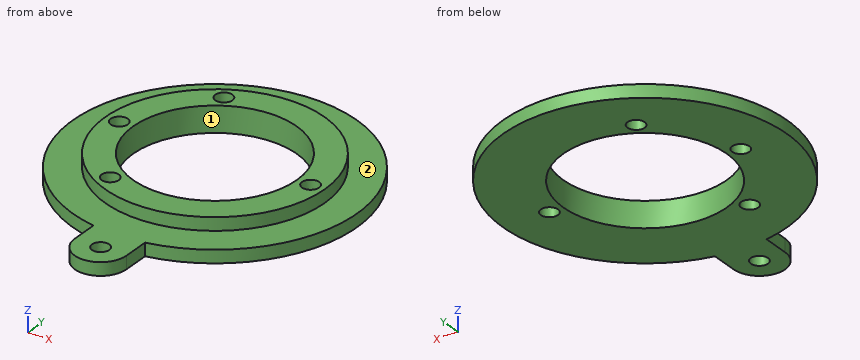
```python
from build123d import *

# Parameters (mm, degrees)
SKETCH010_R     = 25.5
SKETCH010_R_2   = 19
PAD005_DEPTH    = 3
SKETCH011_R     = 19
SKETCH011_R_2   = 2
PAD006_DEPTH    = 3
SKETCH012_R     = 2
POCKET002_DEPTH = 6.001


with BuildPart() as part:
    # Sketch010 → Pad005 (new body)
    with BuildSketch(Plane.XY):
        Circle(SKETCH010_R)
        Circle(SKETCH010_R_2, mode=Mode.SUBTRACT)
    extrude(amount=PAD005_DEPTH)

    # Sketch011 (on Face3 of Pad005) → Pad006 (join)
    with BuildSketch(Plane(origin=(0, 0, 0), x_dir=(1, 0, 0), z_dir=(0, 0, -1))):
        with BuildLine():
            ThreePointArc((-6, 32.449961), (0, -33), (6, 32.449961))
            Line((6, 38.756679), (6, 32.449961))
            ThreePointArc((6, 38.756679), (-1.5e-05, 44.756648), (-6, 38.756648))
            Line((-6, 32.449961), (-6, 38.756648))
        make_face()
        Circle(SKETCH011_R, mode=Mode.SUBTRACT)
        with Locations((0, 38.756648)):
            Circle(SKETCH011_R_2, mode=Mode.SUBTRACT)
    extrude(amount=PAD006_DEPTH)

    # Sketch012 (on Face3 of Pad006) → Pocket002 (cut, through all)
    with BuildSketch(Plane.XY.offset(3)):
        with Locations((-22.25, 0)):
            Circle(SKETCH012_R)
        with Locations((22.25, 0)):
            Circle(SKETCH012_R)
        with Locations((-11.125, 19.269065)):
            Circle(SKETCH012_R)
        with Locations((-11.125, -19.269065)):
            Circle(SKETCH012_R)
    extrude(amount=-POCKET002_DEPTH, mode=Mode.SUBTRACT)


solid = part.part
```
Verification items for the finished model (mm, model axes). Face numbers are marked on the shaded views. Give positions to 0.01 mm unless a question says otherwise; leave off trailing zeros. Order: outer loops, then holes, each group sorted by start corner. A loop starts at its lowest first (then second) coordinate and runs counter-clockwise, first axis right, second up. Notation, with made-up numbers: (78.25, 29) -> (127.25, 29) arc R15 cw to (127.25, 36) -> close; hole circle Ø9 at (-21.75, 50.25). An arc over 180 degrees is marked (long way). One line per item, written item: value.
(1) Sectioned sample at A-A on x = 0. Record the cut outline in (y, z), then the cut area to 3 significant figures.
Final values:
outline: (-44.76, -3) -> (-40.76, -3) -> (-40.76, 0) -> (-44.76, 0) -> close; (-36.76, -3) -> (-19, -3) -> (-19, 3) -> (-25.5, 3) -> (-25.5, 0) -> (-36.76, 0) -> close; (19, -3) -> (33, -3) -> (33, 0) -> (25.5, 0) -> (25.5, 3) -> (19, 3) -> close
area: 146 mm^2
(2) Sectioned sample at C-C on x = 18. Record the cut outline in (y, z), then the cut area to 3 significant figures.
Final values:
outline: (-27.66, -3) -> (-6.08, -3) -> (-6.08, 3) -> (-18.06, 3) -> (-18.06, 0) -> (-27.66, 0) -> close; (6.08, -3) -> (27.66, -3) -> (27.66, 0) -> (18.06, 0) -> (18.06, 3) -> (6.08, 3) -> close
area: 201 mm^2
(3) Sectioned sample at B-B on y = 0. Record the cut outline in (x, z).
Final values:
outline: (-33, -3) -> (-24.25, -3) -> (-24.25, 3) -> (-25.5, 3) -> (-25.5, 0) -> (-33, 0) -> close; (-20.25, -3) -> (-19, -3) -> (-19, 3) -> (-20.25, 3) -> close; (19, -3) -> (20.25, -3) -> (20.25, 3) -> (19, 3) -> close; (24.25, -3) -> (33, -3) -> (33, 0) -> (25.5, 0) -> (25.5, 3) -> (24.25, 3) -> close
(4) Draft check along X on the marked faces 1 and 2. Enter one of: pulls with the +X half, pulls with the -X half, needs draft (parallel to the pull), parting line crosses it, or undercut.
Final values:
face 1: undercut
face 2: needs draft
(5) Scan lines: line 1 along Z through (x, y) = (22, 15.5); line 2 along Y through (x, z) = (8, -0.2); line 3 along X through (y, z) = (8, 1.25). Record each from-to range of solid material in increasing order. Write a range as [from, to].
Final values:
line 1: [-3, 0]
line 2: [-32.02, -17.23], [17.23, 32.02]
line 3: [-24.21, -17.23], [17.23, 24.21]
(6) Sectioned sample at D-D on z = -2.1. Record the cut outline in (x, y) (3 decimals), then the cut area to 3 significant figures.
Final values:
outline: (-6, -38.757) arc R6 ccw to (6, -38.757) -> (6, -32.45) arc R33 ccw (long way) to (-6, -32.45) -> close; hole circle Ø4 at (-22.25, 0); hole circle Ø38 at (0, 0); hole circle Ø4 at (-11.125, -19.269); hole circle Ø4 at (-11.125, 19.269); hole circle Ø4 at (0, -38.757); hole circle Ø4 at (22.25, 0)
area: 2,350 mm^2
(7) Gauge pin test, flat ends, axial feed: pin 1 (0.9 mm diameter, centred on y = -36, z = -1, fed in from +X); pin 2 (3.5 mm diameter, centred on x = -11.12, y = 19.27, fed in from +Z); pin 3 (1.5 mm diameter, centred on x = 23, z = -1.5, fed in from +Y); pin 4 (0.9 mm diameter, centred on y = -35, z = -1, fed in from -X). Record the tip position at first contact, or that the pin passes through.
Final values:
pin 1: x = 6
pin 2: through
pin 3: y = 24.37
pin 4: x = -6
